Part model, mm, in its own coordinate system. Coordinates: 2 decimals unless noted, no trailing zeros. Order: outer loops, then holes, each group sorted by start corner. A loop starts at its lowest first (then second) coordinate and runs counter-clockwise, first axis right, second up. Notation, with made-up numbers: (50, 16.5) - (107, 16.5) arc R32 cw to (107, 52.5) - close; hole circle Ø11 at (-6, -34). An arc over 180 degrees is marked (long way). Use a Markdown table: item, result. Add a question column.
1) Wall check: L1, parallel to Z at x = 14.75, y = 0.1; L2, parallel to Z at x = 8, y = 0.65; L3, parallel to Y at x = 3.75, z = 0.8. Give the ranges that are in metal, low to high. Write a range as [from, to].
2) Saw through at A-A on x = 4.75. List the corners of the cut face in (y, z).
3) Drop flat-ended pins along their axis: P1, Ø1, axis at x = 15, y = -1, coming from the +Z side; P2, Ø1, axis at x = 11.5, y = -1, coming from the -Z side. Give the stop position or say it passes through.
Autodesk Inventor part; units mm, degrees
ref_plane "YZ Plane" through (0, 0, 0) normal (1, 0, 0) x (0, 1, 0)
ref_plane "XZ Plane" through (0, 0, 0) normal (0, 1, 0) x (-1, 0, 0)
ref_plane "XY Plane" through (0, 0, 0) normal (0, 0, 1) x (1, 0, 0)
sketch "Skizze" plane through (0, 0, 0) normal (1, 0, 0) x (0, 1, 0)
  circle A0 centre (0, 0) radius 1.5
  dimension "d1" = 3
extrude "Körper" add sketch "Skizze" along normal blind 20
chamfer "Fase1" distance 0.5 angle 15 1 edges at (0, -1.5, 0) measured on face at (13.3333, 1.4806, -0.2406)
chamfer "Fase2" distance 0.5 angle 15 1 edges at (20, -1.5, 0) measured on face at (13.5, 1.4951, -0.1207)
equation "\"d1\" = NND"
equation "\"d2\" = NLG"
equation "\"d4\" = PHH"
equation "\"d5\" = FAWI"
equation "\"d11\" = PHH"
equation "\"d8\" = PHH"
equation "\"d9\" = FAWI"
equation "\"d12\" = PHH"
equation "\"NND\" = 3"
equation "\"NLG\" = 20"
equation "\"PHH\" = 0.5"
equation "\"FAWI\" = 15deg"
equation "\"KAH\" = 0"
properties part number "ISO 2338 - 3 m6 x 20" material "Edelstahl, austenitisch"
Results are:
| question | item | result |
|---|---|---|
| 1 | L1 | [-1.5, 1.5] |
| 1 | L2 | [-1.35, 1.35] |
| 1 | L3 | [-1.27, 1.27] |
| 2 | outline | circle Ø3 at (0, 0) |
| 3 | P1 | z = 1.41 |
| 3 | P2 | z = -1.41 |
